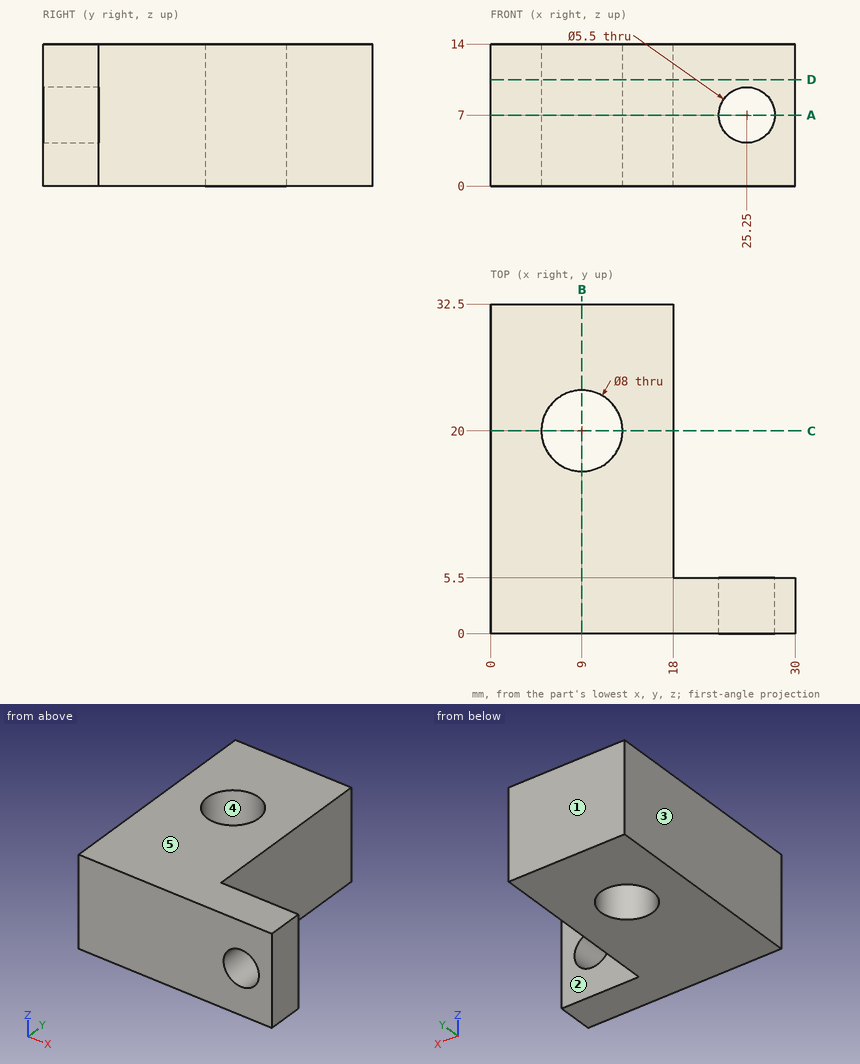
Study the drawing (mm; zero at the part's minimum x, y, z) and answer. A direction names the side the tool comes from. Round coordinates to 2 decimals unless told otherwise and drop trailing zeros. Loops run counter-clockwise (first coordinate to the right, second up) from the corner with the lowest first, then second, coordinate; pieces in that order, holes last. Notation, with made-up numbers: M 88,58 L 93,58 A11 ccw 93,68 Z; hole C 32,-31.5 d7. An arc over 180 degrees is marked long. One line per question, with ' | ' between items.
Q1. Find section D-D, the plane z = 10.5. Give the vertices of the cut face in (x, y).
Conclusion:
outline: M 0,0 L 30,0 L 30,5.5 L 18,5.5 L 18,32.5 L 0,32.5 Z; hole C 9,20 d8
Q2. Each of these flat-tipped pins is pushed along its axis until it touches: pin 1 Ø2 at (x, z) = (22, 6) entering from +Y; pin 2 Ø5 at (y, z) = (13.5, 7) entering from +X. Where does it stop, or does it pass through?
Conclusion:
pin 1: stops at y = 5.5 | pin 2: stops at x = 18
Q3. Find section C-C, the plane y = 20. Give the vertices of the cut face in (x, z), then the cut area to 3 significant figures.
Conclusion:
outline: M 0,0 L 5,0 L 5,14 L 0,14 Z; M 13,0 L 18,0 L 18,14 L 13,14 Z | area: 140 mm2
Q4. Consider line 1 along Y through (x, z) = (9, 8.25); line 2 along X through (y, z) = (3.3, 7); line 3 along Y through (x, z) = (18.5, 13). Determine where each line is inside the solid, lowest interval first. Write a range as from..to.
Conclusion:
line 1: y = 0..16, 24..32.5 | line 2: x = 0..22.5, 28..30 | line 3: y = 0..5.5
Q5. Find section B-B, the plane x = 9. Give the vertices of the cut face in (y, z).
Conclusion:
outline: M 0,0 L 16,0 L 16,14 L 0,14 Z; M 24,0 L 32.5,0 L 32.5,14 L 24,14 Z
Q6. Find section A-A, the plane z = 7. Give the vertices of the cut face in (x, y), then the cut area to 3 significant figures.
Conclusion:
outline: M 0,0 L 22.5,0 L 22.5,5.5 L 18,5.5 L 18,32.5 L 0,32.5 Z; M 28,0 L 30,0 L 30,5.5 L 28,5.5 Z; hole C 9,20 d8 | area: 570 mm2
Q7. A tool of negligible diameter and unlimited length cuts with its end or side. For the marked faces 1 and 2, from which of +Z, -Z, +X, -X, +Y, -Y can it reach the whole face along a straight path? Write none if from no direction.
Conclusion:
face 1: +Z, -Z, +X, -X, +Y | face 2: +Z, -Z, +X, +Y
Q8. The mould has two halves that part along X. Classify the marked faces 3, 4 and 5: +X half, -X half, draft (parallel to the pull), parting line (faces both ways), or undercut.
Conclusion:
face 3: -X half | face 4: undercut | face 5: draft
